Build history of the part. All positions in model axes, mm. Face numbers are marked on the shaded views. A direction names the side the tool comes from. Round coordinates to 2 decimals unless told otherwise and drop trailing zeros. Loops run counter-clockwise (first coordinate to the right, second up) from the corner with the lowest first, then second, coordinate; pieces in that order, holes last.
from build123d import *

# Parameters (mm, degrees)
F1_DEPTH = 4
F2_W     = 2
F2_H     = 5
F2_W_2   = 5
F2_H_2   = 2
F3_DEPTH = 6
F4_R     = 1.99999
F5_W     = 4
F5_H     = 1
F6_DEPTH = 25
F7_R     = 1
F8_W     = 4
F8_H     = 1
F9_DEPTH = 25


# Not quite as in the source:
# - a fillet or chamfer is up to 0.001 mm smaller than in the source, because OpenCascade refuses the exact size


with BuildPart() as f1:
    # F0 (on Top) → F1 (new body)
    with BuildSketch(Plane.XY):
        Polygon((8, -8), (8, 22), (0, 22), (0, 0), (-22, 0), (-22, -8), align=None)
    extrude(amount=F1_DEPTH)

    # F2 (on face) → F3 (join)
    with BuildSketch(Plane.XY.offset(4)):
        with Locations((1, 12.5)):
            Rectangle(F2_W, F2_H)
        with Locations((7, 12.5)):
            Rectangle(F2_W, F2_H)
        with Locations((-12.5, -1)):
            Rectangle(F2_W_2, F2_H_2)
        with Locations((-12.5, -7)):
            Rectangle(F2_W_2, F2_H_2)
    extrude(amount=F3_DEPTH)

    # F4 (radius 2 in the source; OpenCascade refuses exactly that, so slightly less here)
    f4_edges = [f1.edges().sort_by_distance(p)[0] for p in [
        (1, 15, 4),
        (2, 12.5, 4),
        (7, 15, 4),
        (-12.5, -6, 4),
        (-10, -7, 4),
        (1, 10, 4),
        (7, 10, 4),
        (6, 12.5, 4),
        (-15, -7, 4),
        (0, 0, 2),
        (8, -8, 2),
        (-15, -1, 4),
        (-12.5, -2, 4),
        (-10, -1, 4),
        (8, 22, 2),
        (0, 22, 2),
        (-22, -8, 2),
        (-22, 0, 2),
    ]]
    fillet(f4_edges, radius=F4_R)

    # F5 (on face) → F6 (cut)
    with BuildSketch(Plane.XZ.offset(8)):
        with Locations((-5, 0.5)):
            Rectangle(F5_W, F5_H)
    extrude(amount=-F6_DEPTH, mode=Mode.SUBTRACT)

    # F7
    f7_edges = [f1.edges().sort_by_distance(p)[0] for p in [
        (-5, -8, 1),
        (-5, 0, 1),
    ]]
    fillet(f7_edges, radius=F7_R)

    # F8 (on face) → F9 (cut)
    with BuildSketch(Plane.YZ.offset(8)):
        with Locations((5, 0.5)):
            Rectangle(F8_W, F8_H)
    extrude(amount=-F9_DEPTH, mode=Mode.SUBTRACT)


solid = f1.part
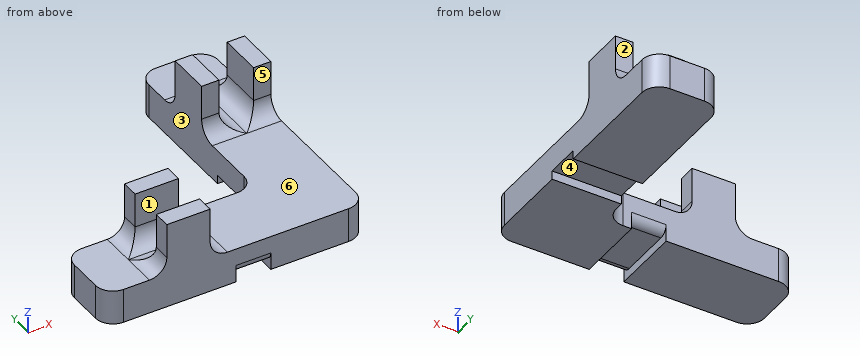
(1) Slice it at D-D on z = 4.75. List the corners of the cut face in (x, y).
Responses:
outline: (-15.44, -8) - (-9.56, -8) - (-9.56, -5.56) - (-15.44, -5.56) - close; (-15.44, -2.44) - (-9.56, -2.44) - (-9.56, 0) - (-15.44, 0) - close; (0, 9.56) - (2.44, 9.56) - (2.44, 15.44) - (0, 15.44) - close; (5.56, 9.56) - (8, 9.56) - (8, 15.44) - (5.56, 15.44) - close
(2) Which spindle directions (+Z, -Z, +X, -X, +Y, -Y) get a long thin tool onto all of the face, cutting with end or side? Do the marked faces 4, 5 and 6. Say none if no direction does.
Responses:
face 4: -Z, +X, -X
face 5: +Z, +X, -X, -Y
face 6: +Z, +X, -Y
(3) Probe line 1 (Y direction, x = -4.75, z = 3); line 2 (Z direction, x = 5.75, y = -5); line 3 (X direction, y = 16.5, z = 2.75). List the from-to ranges inside material, lowest first.
Responses:
line 1: y = -8 to 0
line 2: z = 0 to 4
line 3: x = 0 to 8
(4) Slice it at A-A on z = 8. List the corners of the cut face in (x, y).
Responses:
outline: (-15, -8) - (-10, -8) - (-10, -6) - (-15, -6) - close; (-15, -2) - (-10, -2) - (-10, 0) - (-15, 0) - close; (0, 10) - (2, 10) - (2, 15) - (0, 15) - close; (6, 10) - (8, 10) - (8, 15) - (6, 15) - close
(5) Pull direction Y, two halves, no side cores. Call the marked faces 1, 2 and 3: +Y half, -Y half, draft (parallel to the pull), parting line (faces both ways), or undercut.
Responses:
face 1: undercut
face 2: +Y half
face 3: draft
(6) Pin check, flat tips, straight feed: P1, Ø0.6, axis at y = -1, z = 7.5, coming from the -X side; P2, Ø3, axis at x = 5, y = 7, coming from the +Z side; P3, Ø3, axis at x = -5, y = -5.5, coming from the -Z side. Stop position of each tip, or through.
Responses:
P1: stops at x = -15
P2: stops at z = 4.06
P3: stops at z = 1
